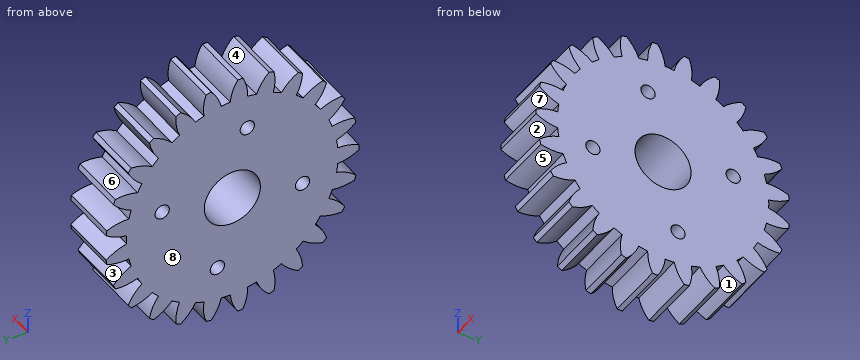
from build123d import *

# Parameters (mm, degrees)
BASPROSKE_W        = 6
BASPROSKE_H        = 13.5
TOOTHCUT_DEPTH     = 21.012496096
TEETHCUTS_COUNT    = 25
TEETHCUTS_ANGLE    = 345.6
BORSKE_R           = 2.5
BORE_DEPTH         = 50.0000508
SKETCH1_R          = 0.762
SKETCH1_R_2        = 2.9845
SKETCH1_R_3        = 2.5
CUT_EXTRUDE1_DEPTH = 149.550528118


with BuildPart() as part:
    # BasProSke → Base-Revolve (revolve)
    with BuildSketch(Plane(origin=(0, 0, 0), x_dir=(1, 0, 0), z_dir=(0, 1, 0)), mode=Mode.PRIVATE) as base_revolve_sk:
        with Locations((3, 6.75)):
            Rectangle(BASPROSKE_W, BASPROSKE_H)
    revolve(base_revolve_sk.sketch.rotate(Axis((-10, 0, 0), (1, 0, 0)), 180), axis=Axis((-10, 0, 0), (1, 0, 0)))

    # TooCutSke → ToothCut (cut, through all)
    with BuildSketch(Plane(origin=(0, 0, 0), x_dir=(0, 0, -1), z_dir=(1, 0, 0))):
        with BuildLine():
            ThreePointArc((0.480087995, 11.238750665), (0, 11.249), (-0.480087995, 11.238750665))
            ThreePointArc((-0.480087995, 11.238750665), (-0.821124963, 12.40220054), (-1.432168974, 13.449361962))
            ThreePointArc((-1.432168974, 13.449361962), (0, 13.5254), (1.432168974, 13.449361962))
            ThreePointArc((1.432168974, 13.449361962), (0.821124963, 12.40220054), (0.480087995, 11.238750665))
        make_face()
    toothcut = extrude(amount=TOOTHCUT_DEPTH, mode=Mode.SUBTRACT)

    # TeethCuts: ToothCut ×25 about axis
    teethcuts_axis = Axis((-10, 0, 0), (1, 0, 0))
    for i in range(1, TEETHCUTS_COUNT):
        add(toothcut.rotate(teethcuts_axis, i * TEETHCUTS_ANGLE / (TEETHCUTS_COUNT - 1)), mode=Mode.SUBTRACT)

    # BorSke → Bore (cut, symmetric)
    with BuildSketch(Plane(origin=(0, 0, 0), x_dir=(0, 0, -1), z_dir=(1, 0, 0))):
        with Locations(Location((0, 0, 0), (0, 0, 180))):
            Circle(BORSKE_R)
    extrude(amount=BORE_DEPTH, both=True, mode=Mode.SUBTRACT)

    # Sketch1 → Cut-Extrude1 (cut, through all)
    # profile 1 of 5: a face of its own
    with BuildSketch(Plane(origin=(0, -120.077012647, 51.383248755), x_dir=(0, 0.18176265719649715, 0.9833424309206171), z_dir=(-1, 0, 0))):
        with Locations(Location((-21.651272984, 124.49267918, 0), (0, 0, 349.527553538))):
            Circle(SKETCH1_R)
    # profile 2 of 5: a face of its own
    with BuildSketch(Plane(origin=(0, -120.077012647, 51.383248755), x_dir=(0, 0.18176265719649715, 0.9833424309206171), z_dir=(-1, 0, 0))):
        with Locations(Location((-25.778113688, 134.466916212, 0), (0, 0, 349.527553538))):
            Circle(SKETCH1_R)
    # profile 3 of 5: a face of its own
    with BuildSketch(Plane(origin=(0, -120.077012647, 51.383248755), x_dir=(0, 0.18176265719649715, 0.9833424309206171), z_dir=(-1, 0, 0))):
        with Locations(Location((-35.752350721, 130.340075507, 0), (0, 0, 349.527553538))):
            Circle(SKETCH1_R)
    # profile 4 of 5: a face of its own
    with BuildSketch(Plane(origin=(0, -120.077012647, 51.383248755), x_dir=(0, 0.18176265719649715, 0.9833424309206171), z_dir=(-1, 0, 0))):
        with Locations(Location((-31.625510016, 120.365838475, 0), (0, 0, 349.527553538))):
            Circle(SKETCH1_R)
    # profile 5 of 5: a face of its own
    with BuildSketch(Plane(origin=(0, -120.077012647, 51.383248755), x_dir=(0, 0.18176265719649715, 0.9833424309206171), z_dir=(-1, 0, 0))):
        with Locations(Location((-28.701811852, 127.416377343, 0), (0, 0, 349.527553538))):
            Circle(SKETCH1_R_2)
        with Locations((-28.701811852, 127.416377343)):
            Circle(SKETCH1_R_3, mode=Mode.SUBTRACT)
    extrude(amount=-CUT_EXTRUDE1_DEPTH, mode=Mode.SUBTRACT)


solid = part.part
The listing builds one solid part. Answer for the finished solid, in the listing's coordinates (mm). Face numbers are marked on the shaded views. A direction names the side the tool comes from. Give positions to 0.01 mm unless a question says otherwise; leave off trailing zeros. One line per question, with ' | ' between items. Start each with the question number.
1. Given P1, Ø1, axis at x = 1, z = -5, coming from the +Y side, flat-ended and moving along its own axis, determine where the tip first touches the part or whether it passes through.
2. Section A-A, the plane x = 5.55 is taken. Count the separate pieces of the cut face and the enclosed holes in it, then the cut area to 3 significant figures.
3. Straight lines are drawn through the part: line 1 (Z direction, x = 5.35, y = 12); line 2 (Y direction, x = 1.25, z = 12); line 3 (Y direction, x = 4.35, z = 10.5). For each, find the intervals that lie inside material, in ascending order.
4. Determine the mould class of the marked faces 6, 7 and 8 for opening direction Y: +Y half, -Y half, draft (parallel to the pull), parting line (faces both ways), or undercut.
5. For the marked faces 1, 2, 3, 4 and 5, determine the directions among +Z, -Z, +X, -X, +Y, -Y from which every point of the face is accessible in a straight line to the end or side of a thin tool.
Result:
1) P1: stops at y = 12.65
2) separate pieces: 1 | enclosed holes: 5 | area: 442 mm2
3) line 1: z = -5.27 to -4.04, -2.32 to -0.67, 0.67 to 2.32, 4.04 to 5.27 | line 2: y = -4.53 to -3.11, -1.58 to 0.09, 1.45 to 3.06, 5.07 to 6.01 | line 3: y = -7.38 to -5.65, -4.38 to 5.87, 8.19 to 8.49
4) face 6: undercut | face 7: -Y half | face 8: draft
5) face 1: -Z, +X, -X | face 2: +X, -X, -Y | face 3: +X, -X, +Y | face 4: +Z, +X, -X | face 5: +X, -X
